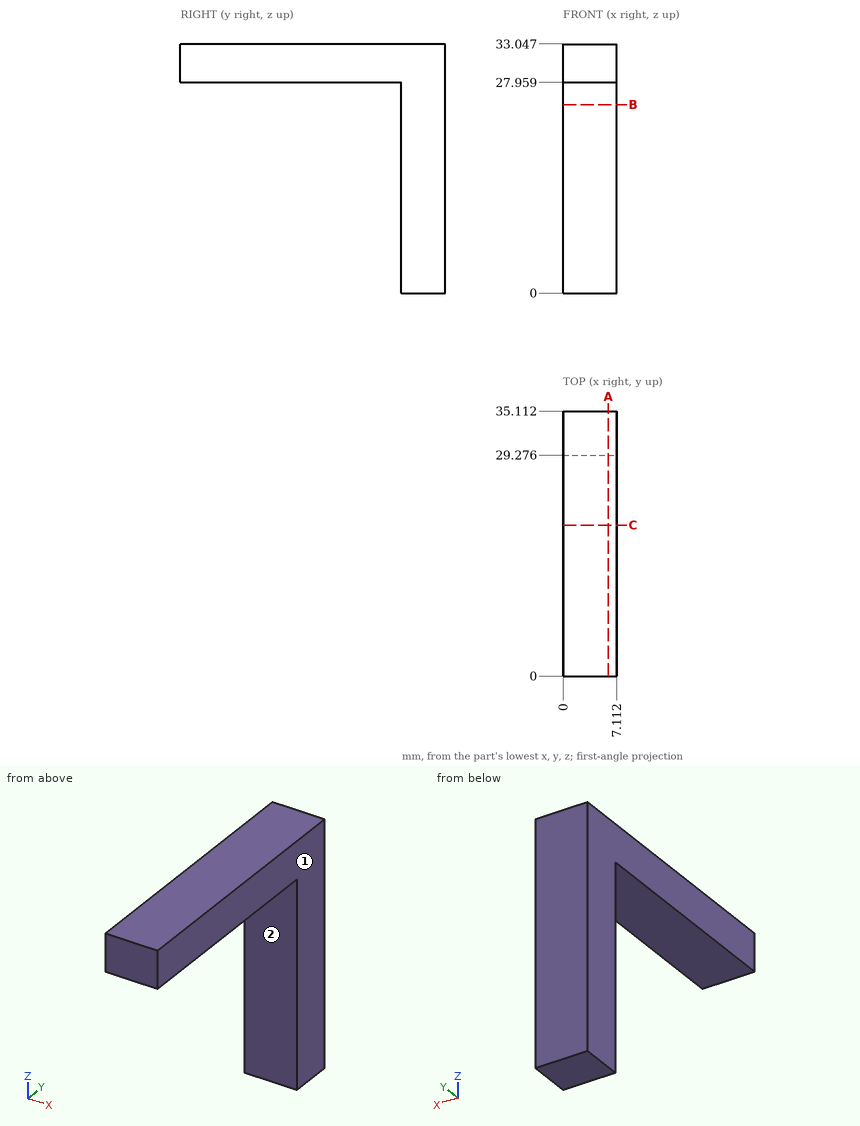
Answer from the drawing. Dimensions are ordinates in mm from the lowest x, y and z of the part. A direction names the side the tool comes from. Round coordinates to 2 decimals unless told otherwise and drop trailing zeros. Loops run counter-clockwise (first coordinate to the right, second up) from the corner with the lowest first, then second, coordinate; pieces in that order, holes last.
1) A cutting plane is placed at B-B on z = 25. Determine the outline of the cut face in (x, y), plus the area to 3 significant figures.
Outcome:
outline: (0, 29.28) - (7.11, 29.28) - (7.11, 35.11) - (0, 35.11) - close
area: 41.5 mm2
2) Given P1, Ø3.5, axis at x = 3.5, y = 15, coming from the -Z side, flat-ended and moving along its own axis, determine where the tip first touches the part or whether it passes through.
Outcome:
P1: stops at z = 27.96
3) Consider line 1 (Z direction, x = 1.25, y = 3); line 2 (Y direction, x = 6.25, z = 22). Determine where each line is inside the solid, lowest interval first.
Outcome:
line 1: z = 27.96 to 33.05
line 2: y = 29.28 to 35.11
4) For the marked faces 1 and 2, determine the directions among +Z, -Z, +X, -X, +Y, -Y from which every point of the face is accessible in a straight line to the end or side of a thin tool.
Outcome:
face 1: +Z, -Z, +X, +Y, -Y
face 2: -Z, +X, -X, -Y
5) A cutting plane is placed at A-A on x = 6. Determine the outline of the cut face in (y, z), plus the area to 3 significant figures.
Outcome:
outline: (0, 27.96) - (29.28, 27.96) - (29.28, 0) - (35.11, 0) - (35.11, 33.05) - (0, 33.05) - close
area: 342 mm2
6) A cutting plane is placed at C-C on y = 20. Determine the outline of the cut face in (x, z), plus the area to 3 significant figures.
Outcome:
outline: (0, 27.96) - (7.11, 27.96) - (7.11, 33.05) - (0, 33.05) - close
area: 36.2 mm2
